CAD build for the part. Positions are in the model's coordinates, mm. Face numbers are marked on the shaded views. A direction names the side the tool comes from. Round coordinates to 2 decimals unless told otherwise and drop trailing zeros. Loops run counter-clockwise (first coordinate to the right, second up) from the corner with the lowest first, then second, coordinate; pieces in that order, holes last. Notation, with made-up numbers: M 74.25,77.25 L 126.25,77.25 A27 cw 126.25,106.25 Z; hole C 36,-38.5 d8. An arc over 180 degrees is marked long. Use one line per item in the form item = value.
from build123d import *

# Parameters (mm, degrees)
SKETCH_1_W          = 90
SKETCH_1_H          = 70
SKETCH_1_W_2        = 80
SKETCH_1_H_2        = 60
EXTRUDE_1_DEPTH     = 15
SKETCH_2_R          = 2.5
CUT_EXTRUDE_1_DEPTH = 98.724101428
SKETCH_3_R          = 5
EXTRUDE_3_DEPTH     = 15
SKETCH_5_R          = 2.5
CUT_EXTRUDE_2_DEPTH = 15
SKETCH_13_R         = 5
SKETCH_13_R_2       = 2.5
EXTRUDE_4_DEPTH     = 5


with BuildPart() as part:
    # 草图1 → 凸台-拉伸1 (new body)
    with BuildSketch(Plane(origin=(0, 0, 0), x_dir=(1, 0, 0), z_dir=(0, 1, 0))):
        with Locations((40, 0)):
            Rectangle(SKETCH_1_W, SKETCH_1_H)
        with Locations((40, 0)):
            Rectangle(SKETCH_1_W_2, SKETCH_1_H_2, mode=Mode.SUBTRACT)
    extrude(amount=EXTRUDE_1_DEPTH)

    # 草图2 → 切除-拉伸1 (cut, through all)
    with BuildSketch(Plane(origin=(85, 0, 0), x_dir=(0, 0, -1), z_dir=(1, 0, 0))):
        with Locations((20, 7.5)):
            Circle(SKETCH_2_R)
        with Locations(Location((-20, 7.5, 0), (0, 0, 180))):
            Circle(SKETCH_2_R)
    extrude(amount=-CUT_EXTRUDE_1_DEPTH, mode=Mode.SUBTRACT)

    # 草图3 → 凸台-拉伸3 (add)
    with BuildSketch(Plane(origin=(0, 15, 0), x_dir=(1, 0, 0), z_dir=(0, 1, 0))):
        with Locations((85, 35)):
            Circle(SKETCH_3_R)
        with Locations((85, -35)):
            Circle(SKETCH_3_R)
        with Locations((-5, -35)):
            Circle(SKETCH_3_R)
        with Locations((-5, 35)):
            Circle(SKETCH_3_R)
    extrude(amount=-EXTRUDE_3_DEPTH)

    # 草图5 → 切除-拉伸2 (cut)
    with BuildSketch(Plane(origin=(0, 15, 0), x_dir=(1, 0, 0), z_dir=(0, 1, 0))):
        with Locations(Location((-5, -35, 0), (0, 0, 270))):
            Circle(SKETCH_5_R)
        with Locations(Location((-5, 35, 0), (0, 0, 270))):
            Circle(SKETCH_5_R)
        with Locations(Location((85, 35, 0), (0, 0, 270))):
            Circle(SKETCH_5_R)
        with Locations(Location((85, -35, 0), (0, 0, 270))):
            Circle(SKETCH_5_R)
    extrude(amount=-CUT_EXTRUDE_2_DEPTH, mode=Mode.SUBTRACT)

    # 草图13 → 凸台-拉伸4 (add)
    # profile 1 of 4: a face of its own
    with BuildSketch(Plane.XZ):
        with Locations(Location((85, -35, 0), (0, 0, 90))):
            Circle(SKETCH_13_R)
        with Locations(Location((85, -35, 0), (0, 0, 90))):
            Circle(SKETCH_13_R_2, mode=Mode.SUBTRACT)
    # profile 2 of 4: a face of its own
    with BuildSketch(Plane.XZ):
        with Locations(Location((85, 35, 0), (0, 0, 270))):
            Circle(SKETCH_13_R)
        with Locations(Location((85, 35, 0), (0, 0, 90))):
            Circle(SKETCH_13_R_2, mode=Mode.SUBTRACT)
    # profile 3 of 4: a face of its own
    with BuildSketch(Plane.XZ):
        with Locations(Location((-5, 35, 0), (0, 0, 90))):
            Circle(SKETCH_13_R)
        with Locations(Location((-5, 35, 0), (0, 0, 90))):
            Circle(SKETCH_13_R_2, mode=Mode.SUBTRACT)
    # profile 4 of 4: a face of its own
    with BuildSketch(Plane.XZ):
        with Locations(Location((-5, -35, 0), (0, 0, 90))):
            Circle(SKETCH_13_R)
        with Locations(Location((-5, -35, 0), (0, 0, 90))):
            Circle(SKETCH_13_R_2, mode=Mode.SUBTRACT)
    extrude(amount=EXTRUDE_4_DEPTH)


solid = part.part
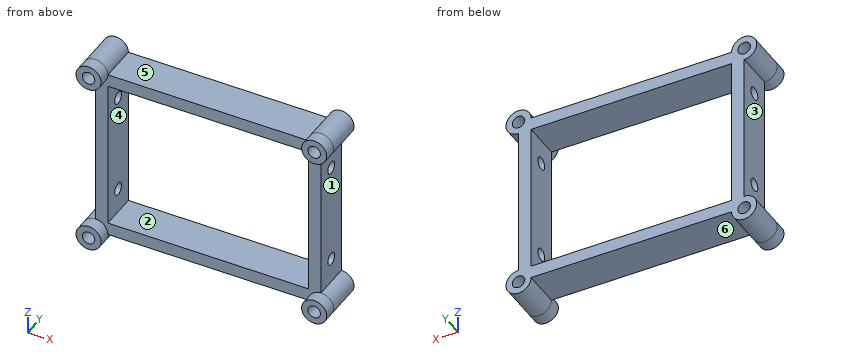
1. Drop flat-ended pins along their axis: P1, Ø1.5, axis at y = 4.5, z = -3, coming from the +X side; P2, Ø1, axis at x = 46.5, y = 11.5, coming from the +Z side; P3, Ø8, axis at y = 7.5, z = 20, coming from the -X side. Give the stop position or say it passes through.
Completed:
P1 = 85
P2 = 35
P3 = -5
2. Cut at A-A on y = -2.75. Write the cut outline in (x, z), and give its area (3 significant figures).
Completed:
outline = C -5,-35 d10; C -5,35 d10; C 85,-35 d10; C 85,35 d10; hole C -5,-35 d5; hole C -5,35 d5; hole C 85,-35 d5; hole C 85,35 d5
area = 236 mm2
3. Cut at C-C on x = 13.5. Write the cut outline in (y, z).
Completed:
outline = M 0,-35 L 15,-35 L 15,-30 L 0,-30 Z; M 0,30 L 15,30 L 15,35 L 0,35 Z
4. Pull direction X, two halves, no side cores. Call the marked faces 1, 2 and 3: +X half, -X half, draft (parallel to the pull), parting line (faces both ways), or undercut.
Completed:
face_1 = +X half
face_2 = undercut
face_3 = -X half
5. Probe line 1 along X through (y, z) = (-1.1, -35); line 2 along X through (y, z) = (3.5, 22); line 3 along Z through (x, y) = (43.5, 2.25). List the from-to ranges inside material, lowest first. Write a range as from..to.
Completed:
line_1 = -10..-7.5, -2.5..0, 80..82.5, 87.5..90
line_2 = -5..0, 80..85
line_3 = -35..-30, 30..35
6. Cut at B-B on z = -3. Write the cut outline in (x, y), and give its area (3 significant figures).
Completed:
outline = M -5,0 L 0,0 L 0,15 L -5,15 Z; M 80,0 L 85,0 L 85,15 L 80,15 Z
area = 150 mm2
7. Cut at D-D on z = 20. Write the cut outline in (x, y), and give its area (3 significant figures).
Completed:
outline = M -5,0 L 0,0 L 0,5 L -5,5 Z; M -5,10 L 0,10 L 0,15 L -5,15 Z; M 80,0 L 85,0 L 85,5 L 80,5 Z; M 80,10 L 85,10 L 85,15 L 80,15 Z
area = 100 mm2
8. Tool access for the marked faces 4, 5 and 6: list every direction of +Z, -Z, +X, -X, +Y, -Y with a clear straight run to the whole face (end or side of a thin tool).
Completed:
face_4 = +Y, -Y
face_5 = +Z, +Y, -Y
face_6 = -Z, +Y, -Y
